from build123d import *

# Parameters (mm, degrees)
SKETCH1_W     = 24
SKETCH1_H     = 9
SKETCH1_W_2   = 17
SKETCH1_H_2   = 5
CHAMFER1_SIZE = 3


with BuildPart() as part:
    # Sketch1 → Revolve1 (revolve)
    with BuildSketch(Plane(origin=(0, 0, 0), x_dir=(0, 0, -1), z_dir=(1, 0, 0)), mode=Mode.PRIVATE) as revolve1_sk:
        with Locations((12, 4.5)):
            Rectangle(SKETCH1_W, SKETCH1_H)
        Polygon((24, 9), (24, 0), (39, 0), (39, 11), (24, 11), align=None)
        Polygon((39, 11), (39, 0), (60, 0), (60, 16), (39, 16), align=None)
        Polygon((60, 16), (60, 0), (70, 0), (70, 14), (70, 22.25), (60, 22.25), align=None)
        Polygon((70, 14), (70, 0), (94.5, 0), (94.5, 9), (94.5, 14), align=None)
        Polygon((94.5, 9), (94.5, 0), (124.5, 0), (124.5, 5), (124.5, 9), align=None)
        with Locations((133, 2.5)):
            Rectangle(SKETCH1_W_2, SKETCH1_H_2)
    revolve(revolve1_sk.sketch.rotate(Axis((0, 0, -60), (0, 0, -1)), 90), axis=Axis((0, 0, -60), (0, 0, -1)))

    # Chamfer1
    chamfer1_edges = [part.edges().sort_by_distance(p)[0] for p in [
        (-9, 0, 0),
    ]]
    chamfer(chamfer1_edges, length=CHAMFER1_SIZE)


solid = part.part
Could you check a few things on this model? Use its own coordinates, in mm. A direction names the side the tool comes from. Round coordinates to 2 decimals unless told otherwise and drop trailing zeros. Loops run counter-clockwise (first coordinate to the right, second up) from the corner with the lowest first, then second, coordinate; pieces in that order, holes last. Notation, with made-up numbers: (-2, 60.25) - (3, 60.25) arc R24 cw to (3, 79.25) - close; hole circle Ø7 at (39, -12.75). An arc over 180 degrees is marked (long way). Write item = value, one per line.
1) I need wall thicknesses on line 1 along Z through (x, y) = (10.5, -17.5); line 2 along Y through (x, z) = (7.5, -105); line 3 along Z through (x, y) = (5, -2). Which ranges of each line are inside material? Lowest first, please. Write a range as from..to.
Computed:
line_1 = -70..-60
line_2 = -4.97..4.97
line_3 = -124.5..0
2) I'm going to push flat-ended pins straight in: P1, Ø8, axis at y = -3, z = -117.5, coming from the -X side; P2, Ø10, axis at x = -7, y = -10.5, coming from the -Z side; P3, Ø5, axis at y = -15.5, z = -23, coming from the -X side; P4, Ø3, axis at y = -3, z = -18, coming from the -X side. Where does each tip first touch, or does it pass through?
Computed:
P1 = -9
P2 = -124.5
P3 = through
P4 = -8.87
3) On a 3-axis mill with a long thin cutter (end or side, diameter ignored), from which of +Z, -Z, +X, -X, +Y, -Y can I reach the whole of each face in a straight line? I mean faces 1 (the flat face through (0, 0, 0)), 2 (the flat face through (0, 15, -70)), 3 (the cylindrical face through (-2.38, 10.74, -31.4)). Say none if no direction works.
Computed:
face_1 = +Z, +X, -X, +Y, -Y
face_2 = -Z
face_3 = +Z
4) Imagine slicing it at D-D (z = -117.5). Please give me the cut outline in (x, y), and give its area (3 significant figures).
Computed:
outline = circle Ø18 at (0, 0)
area = 254 mm2
5) Imagine slicing it at C-C (z = -92). Please give me the cut outline in (x, y).
Computed:
outline = circle Ø28 at (0, 0)
